For this review, take the finished solid that the model builds, in its own axes (mm). A direction names the side the tool comes from. Round coordinates to 2 decimals unless told otherwise and drop trailing zeros. Write each loop counter-clockwise with the first axis right and the second up, starting at its lowest first coordinate (ties: lowest second). Pieces come first, ordered by that corner, then holes. Notation, with made-up numbers: (59, -24.5) - (90, -24.5) arc R17 ccw to (90, -6.5) - close; hole circle Ø1 at (40.25, 67.5). An arc over 180 degrees is marked (long way). One line per item, written item: value. Start each with the question number.
Q1. Mouldability with a two-part tool opening along Y and no side actions: class faces 4 (the face through (-9.699, -9.715, 4.93)), 5 (the face through (-4, 8, 5)), 6 (the face through (2, 2, 0)), 7 (the face through (0, 4, 5)) as +Y half, -Y half, draft (parallel to the pull), parting line (faces both ways), or undercut.
Q2. For probe 1 along Y at (x, z) = (0, 5.25); probe 2 along Y at (x, z) = (5.75, 7); probe 3 along Y at (x, z) = (3.5, 5.75), list the stretches that pass through material, from the lowest coordinate up.
Q3. Tool access review of faces 1 (the face through (9, 3, 5)), 2 (the face through (5.844, -7.684, 4.93)), 3 (the face through (-3, -9, 5)): name each direction out of +Z, -Z, +X, -X, +Y, -Y from which nothing blocks a thin tool from reaching the whole face with its end or side.
Q4. Clearance check with flat-ended pins moving along their axes: pin 1 Ø1.1 at (x, z) = (0.5, 5.5) entering from -Y; pin 2 Ø4 at (y, z) = (-0.5, 6.5) entering from +X. State where each tip first meets the part, or that it passes through.
Q5. Add section A-A on y = 0. Write out the cut boundary in (x, z), and give its area (3 significant figures).
Autodesk Inventor part; units mm, degrees
ref_plane "Start Plane" through (0, 0, 0) normal (0, 0, 1) x (1, 0, 0)
ref_plane "End Plane" through (0, 0, 10) normal (0, 0, 1) x (1, 0, 0)
ref_plane "YZ Plane" through (0, 0, 0) normal (1, 0, 0) x (0, 1, 0)
ref_plane "Start Plane" through (0, 0, 0) normal (0, 0, 1) x (1, 0, 0)
ref_plane "End Plane" through (0, 0, 10) normal (0, 0, 1) x (1, 0, 0)
sketch "Sketch1" plane through (0, 0, 0) normal (0, 0, 1) x (1, 0, 0)
  line L0 (0, 0) -> (2.5, 0) construction
  line L1 (0, 0) -> (0, 2.5) construction
  line L2 (0, 4) -> (0, -4) construction
  line L3 (0, 4) -> (1.7574, 4)
  arc A0 (1.7574, 4) -> (3.1716, 4.5858) centre (1.7574, 6) ccw
  line L4 (3.1716, 4.5858) -> (5.7322, 7.1464)
  line L5 (-4, 0) -> (4, 0) construction
  line L6 (4, 0) -> (4, 1.7574)
  arc A1 (4.5858, 3.1716) -> (4, 1.7574) centre (6, 1.7574) ccw
  line L7 (4.5858, 3.1716) -> (7.1464, 5.7322)
  line L8 (0, 0) -> (10, 10) construction
  line L9 (0, 0) -> (19.6827, 0) construction
  arc A2 (8, 5.3787) -> (7.1464, 5.7322) centre (7.5, 5.3787) ccw
  line L10 (8, 5.3787) -> (8, 3.5)
  arc A3 (8, 3.5) -> (8.5, 3) centre (8.5, 3.5) ccw
  line L11 (8.5, 3) -> (9.5, 3)
  arc A4 (9.5, 3) -> (10, 3.5) centre (9.5, 3.5) ccw
  line L12 (10, 3.5) -> (10, 9)
  line L13 (10, 9) -> (10, 10) construction
  arc A5 (5.7322, 7.1464) -> (5.3787, 8) centre (5.3787, 7.5) ccw
  line L14 (5.3787, 8) -> (3.5, 8)
  arc A6 (3, 8.5) -> (3.5, 8) centre (3.5, 8.5) ccw
  line L15 (3, 8.5) -> (3, 9.5)
  arc A7 (3.5, 10) -> (3, 9.5) centre (3.5, 9.5) ccw
  line L16 (3.5, 10) -> (9, 10)
  arc A8 (10, 9) -> (9, 10) centre (9, 9) ccw
  line L17 (0, 4) -> (-1.7574, 4)
  arc A9 (-3.1716, 4.5858) -> (-1.7574, 4) centre (-1.7574, 6) ccw
  line L18 (-3.1716, 4.5858) -> (-5.7322, 7.1464)
  line L19 (-4, 0) -> (-4, 1.7574)
  arc A10 (-4, 1.7574) -> (-4.5858, 3.1716) centre (-6, 1.7574) ccw
  line L20 (-4.5858, 3.1716) -> (-7.1464, 5.7322)
  arc A11 (-7.1464, 5.7322) -> (-8, 5.3787) centre (-7.5, 5.3787) ccw
  line L21 (-8, 5.3787) -> (-8, 3.5)
  arc A12 (-8.5, 3) -> (-8, 3.5) centre (-8.5, 3.5) ccw
  line L22 (-8.5, 3) -> (-9.5, 3)
  arc A13 (-10, 3.5) -> (-9.5, 3) centre (-9.5, 3.5) ccw
  line L23 (-10, 3.5) -> (-10, 9)
  arc A14 (-5.3787, 8) -> (-5.7322, 7.1464) centre (-5.3787, 7.5) ccw
  line L24 (-5.3787, 8) -> (-3.5, 8)
  arc A15 (-3.5, 8) -> (-3, 8.5) centre (-3.5, 8.5) ccw
  line L25 (-3, 8.5) -> (-3, 9.5)
  arc A16 (-3, 9.5) -> (-3.5, 10) centre (-3.5, 9.5) ccw
  line L26 (-3.5, 10) -> (-9, 10)
  arc A17 (-9, 10) -> (-10, 9) centre (-9, 9) ccw
  line L27 (0, -4) -> (-1.7574, -4)
  arc A18 (-1.7574, -4) -> (-3.1716, -4.5858) centre (-1.7574, -6) ccw
  line L28 (-3.1716, -4.5858) -> (-5.7322, -7.1464)
  arc A19 (-5.7322, -7.1464) -> (-5.3787, -8) centre (-5.3787, -7.5) ccw
  line L29 (-5.3787, -8) -> (-3.5, -8)
  arc A20 (-3, -8.5) -> (-3.5, -8) centre (-3.5, -8.5) ccw
  line L30 (-3, -8.5) -> (-3, -9.5)
  arc A21 (-3.5, -10) -> (-3, -9.5) centre (-3.5, -9.5) ccw
  line L31 (-3.5, -10) -> (-9, -10)
  arc A22 (-10, -9) -> (-9, -10) centre (-9, -9) ccw
  line L32 (-10, -3.5) -> (-10, -9)
  arc A23 (-9.5, -3) -> (-10, -3.5) centre (-9.5, -3.5) ccw
  line L33 (-8.5, -3) -> (-9.5, -3)
  arc A24 (-8, -3.5) -> (-8.5, -3) centre (-8.5, -3.5) ccw
  line L34 (-8, -5.3787) -> (-8, -3.5)
  arc A25 (-8, -5.3787) -> (-7.1464, -5.7322) centre (-7.5, -5.3787) ccw
  line L35 (-4.5858, -3.1716) -> (-7.1464, -5.7322)
  arc A26 (-4.5858, -3.1716) -> (-4, -1.7574) centre (-6, -1.7574) ccw
  line L36 (-4, 0) -> (-4, -1.7574)
  line L37 (3.5, -10) -> (9, -10)
  arc A27 (9, -10) -> (10, -9) centre (9, -9) ccw
  line L38 (10, -3.5) -> (10, -9)
  arc A28 (10, -3.5) -> (9.5, -3) centre (9.5, -3.5) ccw
  line L39 (8.5, -3) -> (9.5, -3)
  arc A29 (8.5, -3) -> (8, -3.5) centre (8.5, -3.5) ccw
  line L40 (8, -5.3787) -> (8, -3.5)
  arc A30 (7.1464, -5.7322) -> (8, -5.3787) centre (7.5, -5.3787) ccw
  line L41 (4.5858, -3.1716) -> (7.1464, -5.7322)
  arc A31 (4, -1.7574) -> (4.5858, -3.1716) centre (6, -1.7574) ccw
  line L42 (4, 0) -> (4, -1.7574)
  line L43 (5.3787, -8) -> (3.5, -8)
  arc A32 (5.3787, -8) -> (5.7322, -7.1464) centre (5.3787, -7.5) ccw
  line L44 (3.1716, -4.5858) -> (5.7322, -7.1464)
  arc A33 (3.1716, -4.5858) -> (1.7574, -4) centre (1.7574, -6) ccw
  line L45 (0, -4) -> (1.7574, -4)
  arc A34 (3.5, -8) -> (3, -8.5) centre (3.5, -8.5) ccw
  line L46 (3, -8.5) -> (3, -9.5)
  arc A35 (3, -9.5) -> (3.5, -10) centre (3.5, -9.5) ccw
  circle A36 centre (0, 0) radius 2.5
  dimension "d1" = 8
  dimension "d2" = 2
  dimension "d3" = 8
  dimension "d4" = 2
  dimension "d5" = 2
  dimension "d7" = 45
  dimension "d8" = 0.5
  dimension "d9" = 0.5
  dimension "d10" = 0.5
  dimension "d12" = 2
  dimension "d17" = 7
  dimension "d18" = 10
  dimension "d19" = 0.5
  dimension "d20" = 1
  dimension "d21" = 0.5
  dimension "d22" = 0.5
  dimension "d23" = 2
  dimension "d24" = 7
  dimension "d25" = 5
extrude "Body" add sketch "Sketch1" along normal up to surface (10 mm away) from surface at 0
sketch "Sketch2" plane through (0, 0, 0) normal (0, 0, 1) x (1, 0, 0)
  line L0 (0, 0) -> (10, 0)
ref_plane "Work Plane3" through (0, 0, 0) normal (0, -1, 0) x (1, 0, 0)
sketch "Sketch3" plane through (0, 0, 0) normal (0, -1, 0) x (1, 0, 0)
  line L0 (-14, 0) -> (14, 0)
  line L1 (-14, 10) -> (14, 10)
  dimension "d33" = 10
equation "\"d1\" = 0.8 * sigma"
equation "\"d2\" = 0.2 * sigma"
equation "\"d3\" = 0.8 * sigma"
equation "\"d4\" = 0.2 * sigma"
equation "\"d5\" = 0.2 * sigma"
equation "\"d8\" = 0.05 * sigma"
equation "\"d9\" = 0.05 * sigma"
equation "\"d10\" = 0.05 * sigma"
equation "\"d12\" = 0.2 * sigma"
equation "\"d17\" = 0.7 * sigma"
equation "\"d18\" = sigma"
equation "\"d19\" = 0.05 * sigma"
equation "\"d20\" = 0.1 * sigma"
equation "\"d21\" = 0.05 * sigma"
equation "\"d22\" = 0.05 * sigma"
equation "\"d23\" = 0.2 * sigma"
equation "\"d24\" = 0.7 * sigma"
equation "\"d25\" = 0.5 * sigma"
equation "\"sigma\" = 1"
equation "\"G_OFFSET_START\" = 0"
equation "\"G_OFFSET_END\" = 0"
equation "\"G_L\" = d33"
properties part number "A3.3-MEM"
Result set:
1. face 4: -Y half
1. face 5: undercut
1. face 6: draft
1. face 7: +Y half
2. probe 1: y = -4 to -2.5, 2.5 to 4
2. probe 2: y = -10 to -7.83, -7.17 to -4.34, 4.34 to 7.17, 7.83 to 10
2. probe 3: y = -10 to -8, -4.91 to 4.91, 8 to 10
3. face 1: +Z, -Z, +X
3. face 2: +Z, -Z
3. face 3: +Z, -Z, -Y
4. pin 1: stops at y = -4
4. pin 2: stops at x = 4.14
5. outline: (-4, 0) - (-2.5, 0) - (-2.5, 10) - (-4, 10) - close; (2.5, 0) - (4, 0) - (4, 10) - (2.5, 10) - close
5. area: 30.0 mm^2
